Solid Edge part; units mm, degrees
sketch "Sketch1" plane through (0, 0, 0) normal (0, 0, 1) x (1, 0, 0)
  line L0 (0, 5.19) -> (0, 3.2255)
  line L1 (0, 3.2255) -> (21.1, 1.75)
  line L2 (21.1, 1.75) -> (30, 1.75)
  line L3 (30, 1.75) -> (30, 4.86)
  arc A0 (30, 4.86) -> (27.36, 7.5) centre (27.36, 4.86) ccw
  line L4 (27.36, 7.5) -> (25.9651, 7.5)
  line L5 (25.9651, 7.5) -> (22.15, 11.3151)
  line L6 (22.15, 11.3151) -> (17, 11.3151)
  line L7 (17, 11.3151) -> (17, 6.6)
  line L8 (17, 6.6) -> (13.2, 6.6)
  line L9 (13.2, 6.6) -> (13.2, 7.5)
  line L10 (13.2, 7.5) -> (12.5301, 10)
  line L11 (12.5301, 10) -> (8, 10)
  line L12 (8, 10) -> (8, 5.19)
  line L13 (8, 5.19) -> (6.4, 5.19)
  line L14 (6.4, 5.19) -> (4.997, 6)
  line L15 (4.997, 6) -> (0.81, 6)
  line L16 (0.81, 6) -> (0, 5.19)
revolve "RevolvedProtrusion1" add sketch "Sketch1" angle 360 about axis through (30, 0, 0) along (-1, 0, 0)
sketch "Sketch2" plane through (13.2, 0, 0) normal (1, 0, 0) x (0, 1, 0)
  line L0 (15, 15) -> (-15, 15)
  line L1 (-15, 15) -> (-15, -15)
  line L2 (-15, -15) -> (15, -15)
  line L3 (15, -15) -> (15, 15)
  arc A0 (0.671, 8.2728) -> (-0.671, 8.2728) centre (0, 0) ccw
  line L4 (-0.671, 8.2728) -> (-6.829, 4.7176)
  arc A1 (-6.829, 4.7176) -> (-7.5, 3.5553) centre (0, 0) ccw
  line L5 (-7.5, 3.5553) -> (-7.5, -3.5553)
  arc A2 (-7.5, -3.5553) -> (-6.829, -4.7176) centre (0, 0) ccw
  line L6 (-6.829, -4.7176) -> (-0.671, -8.2728)
  arc A3 (-0.671, -8.2728) -> (0.671, -8.2728) centre (0, 0) ccw
  line L7 (0.671, -8.2728) -> (6.829, -4.7176)
  arc A4 (6.829, -4.7176) -> (7.5, -3.5553) centre (0, 0) ccw
  line L8 (7.5, -3.5553) -> (7.5, 3.5553)
  arc A5 (7.5, 3.5553) -> (6.829, 4.7176) centre (0, 0) ccw
  line L9 (6.829, 4.7176) -> (0.671, 8.2728)
extrude "ExtrudedCutout_1" cut sketch "Sketch2" against normal blind 5.2
sketch "Sketch3" plane through (17, 0, 0) normal (1, 0, 0) x (0, 1, 0)
  line L0 (15, 15) -> (-15, 15)
  line L1 (-15, 15) -> (-15, -15)
  line L2 (-15, -15) -> (15, -15)
  line L3 (15, -15) -> (15, 15)
  arc A0 (0.671, 8.2728) -> (-0.671, 8.2728) centre (0, 0) ccw
  line L4 (-0.671, 8.2728) -> (-6.829, 4.7176)
  arc A1 (-6.829, 4.7176) -> (-7.5, 3.5553) centre (0, 0) ccw
  line L5 (-7.5, 3.5553) -> (-7.5, -3.5553)
  arc A2 (-7.5, -3.5553) -> (-6.829, -4.7176) centre (0, 0) ccw
  line L6 (-6.829, -4.7176) -> (-0.671, -8.2728)
  arc A3 (-0.671, -8.2728) -> (0.671, -8.2728) centre (0, 0) ccw
  line L7 (0.671, -8.2728) -> (6.829, -4.7176)
  arc A4 (6.829, -4.7176) -> (7.5, -3.5553) centre (0, 0) ccw
  line L8 (7.5, -3.5553) -> (7.5, 3.5553)
  arc A5 (7.5, 3.5553) -> (6.829, 4.7176) centre (0, 0) ccw
  line L9 (6.829, 4.7176) -> (0.671, 8.2728)
extrude "ExtrudedCutout_2" cut sketch "Sketch3" along normal blind 30
sketch "Sketch4" plane through (0, 7.5, 0) normal (0, -1, 0) x (1, 0, 0)
  line L0 (8.6933, -1.9067) -> (8.6933, 1.9067)
  line L1 (8.6933, 1.9067) -> (12.5067, 1.9067)
  line L2 (12.5067, 1.9067) -> (12.5067, -1.9067)
  line L3 (12.5067, -1.9067) -> (8.6933, -1.9067)
  arc A0 (8.9062, -0.3681) -> (9.446, 1.2934) centre (10.6, 0) cw
  line L4 (9.446, 1.2934) -> (9.5245, 1.1854)
  arc A1 (9.5245, 1.1854) -> (9.805, 1.3892) centre (9.9887, 0.8414) ccw
  line L5 (9.805, 1.3892) -> (9.7265, 1.4971)
  arc A2 (9.7265, 1.4971) -> (11.4735, 1.4971) centre (10.6, 0) cw
  line L6 (11.4735, 1.4971) -> (11.395, 1.3892)
  arc A3 (11.395, 1.3892) -> (11.6755, 1.1854) centre (11.2113, 0.8414) ccw
  line L7 (11.6755, 1.1854) -> (11.754, 1.2934)
  arc A4 (11.754, 1.2934) -> (12.2938, -0.3681) centre (10.6, 0) cw
  line L8 (12.2938, -0.3681) -> (12.1669, -0.3268)
  arc A5 (12.1669, -0.3268) -> (12.0597, -0.6565) centre (11.5891, -0.3214) ccw
  line L9 (12.0597, -0.6565) -> (12.1867, -0.6978)
  arc A6 (12.1867, -0.6978) -> (10.7733, -1.7246) centre (10.6, 0) cw
  line L10 (10.7733, -1.7246) -> (10.7733, -1.5912)
  arc A7 (10.7733, -1.5912) -> (10.4267, -1.5912) centre (10.6, -1.04) ccw
  line L11 (10.4267, -1.5912) -> (10.4267, -1.7246)
  arc A8 (10.4267, -1.7246) -> (9.0133, -0.6978) centre (10.6, 0) cw
  line L12 (9.0133, -0.6978) -> (9.1403, -0.6565)
  arc A9 (9.1403, -0.6565) -> (9.0331, -0.3268) centre (9.6109, -0.3214) ccw
  line L13 (9.0331, -0.3268) -> (8.9062, -0.3681)
extrude "ExtrudedCutout_3" cut sketch "Sketch4" along normal blind 0.03
properties part number "SKINTOP ST-M 12x1,5      Art. Nr. 53111000(F=3.5)"
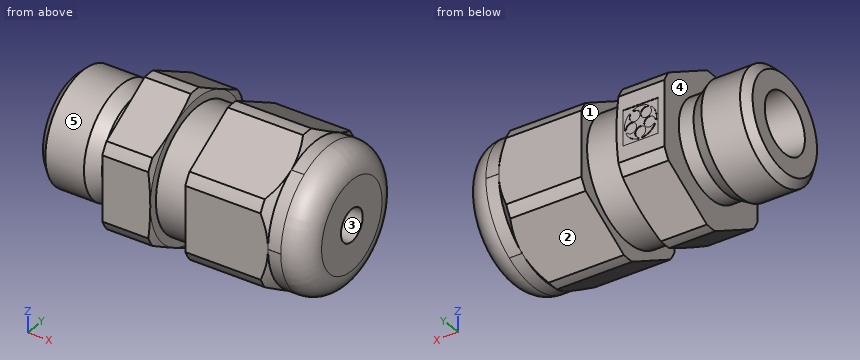
Build history of the part. All positions in model axes, mm. Face numbers are marked on the shaded views. A direction names the side the tool comes from. Round coordinates to 2 decimals unless told otherwise and drop trailing zeros. Loops run counter-clockwise (first coordinate to the right, second up) from the corner with the lowest first, then second, coordinate; pieces in that order, holes last.
Item 1: Which spindle directions (+Z, -Z, +X, -X, +Y, -Y) get a long thin tool onto all of the face, cutting with end or side? Do the marked faces 1 and 2. Say none if no direction does.
Item 2: Saw through at A-A (x = 15). List the corners of the cut face in (y, z).
Item 3: Drill centre lines: line 1 along Y through (x, z) = (23.5, 0); line 2 along Y through (x, z) = (26, -6.5); line 3 along Y through (x, z) = (3.5, 2). Where is each one in solid material? Low to high.
Item 4: Two-plate mould, pull along Z, no slides. Class the marked faces 3, 4 and 5: released by +Z, released by -Z, zero draft, split by the parting line, or undercut.
Item 5: Pin check, flat tips, straight feed: P1, Ø2, axis at y = -0.5, z = 3, coming from the -X side; P2, Ø3, axis at y = 0, z = 0, coming from the +X side; P3, Ø1.5, axis at x = 13, y = -1.5, coming from the +Z side; P4, Ø2, axis at x = 23.5, y = 2.5, coming from the -Z side. Stop position of each tip, or through.
Worked answers:
1. face 1: none
1. face 2: -Z, +X, -X, +Y
2. outline: circle Ø13.2 at (0, 0); hole circle Ø4.35 at (0, 0)
3. line 1: y = -7.5 to -1.75, 1.75 to 7.5
3. line 2: y = -3.74 to 3.74
3. line 3: y = -5.66 to -2.21, 2.21 to 5.66
4. face 3: undercut
4. face 4: zero draft
4. face 5: split by the parting line
5. P1: stops at x = 0
5. P2: passes through
5. P3: stops at z = 8.23
5. P4: stops at z = -7.79
